from build123d import *

# Parameters (mm, degrees)
CUT_EXTRUDE_1_DEPTH = 12
CUT_EXTRUDE_2_DEPTH = 9
CHAMFER_1_SIZE      = 2
FILLET_1_R          = 2


with BuildPart() as part:
    # 草图1 → 旋转1 (revolve)
    with BuildSketch(Plane.XY, mode=Mode.PRIVATE) as revolve_1_sk:
        Polygon((0, 0), (0, 15), (28, 15), (28, 16), (53, 16), (53, 18), (66, 18), (66, 13.5), (68, 13.5), (68, 15), (82, 15), (82, 14), (106, 14), (106, 12), (140, 12), (140, 0), align=None)
    revolve(revolve_1_sk.sketch.rotate(Axis((0, 0, 0), (1, 0, 0)), 90), axis=Axis((0, 0, 0), (1, 0, 0)))

    # 草图2 → 切除-拉伸1 (cut)
    with BuildSketch(Plane.XY.offset(20)):
        with BuildLine():
            Line((113, 4), (130, 4))
            ThreePointArc((130, 4), (134, 0), (130, -4))
            Line((130, -4), (113, -4))
            ThreePointArc((113, -4), (109, 0), (113, 4))
        make_face()
    extrude(amount=-CUT_EXTRUDE_1_DEPTH, mode=Mode.SUBTRACT)

    # 草图3 → 切除-拉伸2 (cut)
    with BuildSketch(Plane.XY.offset(20)):
        with BuildLine():
            Line((34, 5), (46, 5))
            ThreePointArc((46, 5), (51, 0), (46, -5))
            Line((46, -5), (34, -5))
            ThreePointArc((34, -5), (29, 0), (34, 5))
        make_face()
    extrude(amount=-CUT_EXTRUDE_2_DEPTH, mode=Mode.SUBTRACT)

    # 倒角1
    chamfer_1_edges = [part.edges().sort_by_distance(p)[0] for p in [
        (140, 0, -12),
        (0, 0, -15),
    ]]
    chamfer(chamfer_1_edges, length=CHAMFER_1_SIZE)

    # 圆角1
    fillet_1_edges = [part.edges().sort_by_distance(p)[0] for p in [
        (106, 0, -12),
    ]]
    fillet(fillet_1_edges, radius=FILLET_1_R - 0.0001)  # a hair under: the kernel refuses the full size


solid = part.part
Check sheet for the modelled part. Datum: model origin and axes. Units: mm. A direction names the side the tool comes from. Give positions to 0.01 mm unless a question says otherwise; leave off trailing zeros. Loops run counter-clockwise (first coordinate to the right, second up) from the corner with the lowest first, then second, coordinate; pieces in that order, holes last. Notation, with made-up numbers: M -31,31 L -21,31 A24 ccw -21,48 Z; hole C 61.5,-27.75 d9. An arc over 180 degrees is marked long. Use a Markdown table: item, result. Add a question column.
Q1. Scan lines: line 1 along Y through (x, z) = (113.5, 9.5); line 2 along Y through (x, z) = (107.5, 0); line 3 along Z through (x, y) = (80.5, -2.5). Record each from-to range of solid material in increasing order. Write a range as [from, to].
Q2. Sectioned sample at D-D, the plane x = 98. Record the cut outline in (y, z), then the cut area to 3 significant figures.
Q3. Go/stop test with flat-tipped pins: pin 1 (2.5 mm diameter, centred on x = 118.5, z = 9.5, fed in from +Y); pin 2 (6 mm diameter, centred on x = 79, y = -10, fed in from -Z); pin 3 (10 mm diameter, centred on y = 13.5, z = 7.5, fed in from +X). Record where each tip stops, or that it passes through.
Q4. Sectioned sample at C-C, the plane x = 70. Record the cut outline in (y, z), then the cut area to 3 significant figures.
Q5. Sectioned sample at B-B, the plane x = 121.5. Record the cut outline in (y, z).
Q6. Mould release check, pull along Y, two halves, no side actions. Record for faces 6 (the cylindrical face through (134, 0, 10)), 7 (the cylindrical face through (94.2, 12.4, 6.5)), 8 (the flat face through (0, 0, 0)): pulls with the +Y half, pulls with the -Y half, needs draft (parallel to the pull), parting line crosses it, or undercut.
Q7. Tool access check on faces 1 (the cylindrical face through (59.591, -12.165, -13.267)), 2 (the cylindrical face through (40.675, 9.736, -12.697)), 3 (the flat face through (68, -7.85, 11.18)), 4 (the cylindrical face through (123.21, 7.302, -9.523)), 5 (the flat face through (122, -4, 10)). Record the directions out of +Z, -Z, +X, -X, +Y, -Y that give a thin tool (end or side, any length) a straight path to the whole face; none if there is none.
Verdict:
| question | item | result |
|---|---|---|
| 1 | line 1 | [-7.33, -4], [4, 7.33] |
| 1 | line 2 | [-12.06, 12.06] |
| 1 | line 3 | [-14.79, 14.79] |
| 2 | outline | C 0,0 d28 |
| 2 | area | 616 mm^2 |
| 3 | pin 1 | y = 8.71 |
| 3 | pin 2 | z = -13.27 |
| 3 | pin 3 | x = 139.56 |
| 4 | outline | C 0,0 d30 |
| 4 | area | 707 mm^2 |
| 5 | outline | M -4,8 L -4,11.31 A12 ccw long 4,11.31 L 4,8 Z |
| 6 | face 6 | undercut |
| 6 | face 7 | parting line crosses it |
| 6 | face 8 | needs draft |
| 7 | face 1 | +X, -X |
| 7 | face 2 | -X |
| 7 | face 3 | none |
| 7 | face 4 | +X |
| 7 | face 5 | +Z |
